Read the model definition and answer for the solid it produces. Units are mm, in the model's axes. Face numbers are marked on the shaded views. Coordinates: 2 decimals unless noted, no trailing zeros. Order: outer loops, then holes, each group sorted by start corner. A loop starts at its lowest first (then second) coordinate and runs counter-clockwise, first axis right, second up.
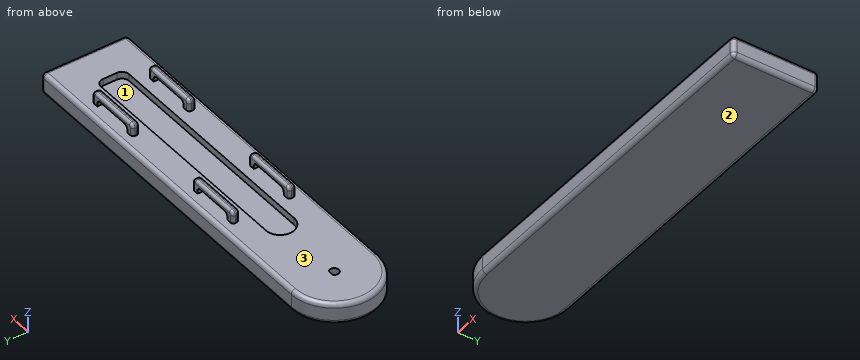
```python
from build123d import *

# Parameters (mm, degrees)
BOSS_EXTRUDE1_DEPTH               = 15
CONG_2_R                          = 3
ENL_V_MAT_EXTRU_3_DEPTH           = 10
BOSS_EXTRU_1_DEPTH                = 5
CONG_3_R                          = 3
CONG_4_R                          = 3
R_P_TITION_LIN_AIRE1_COUNT        = 2
R_P_TITION_LIN_AIRE1_PITCH        = 100
R_P_TITION_LIN_AIRE2_COUNT        = 2
R_P_TITION_LIN_AIRE2_PITCH        = 40
R_P_TITION_LIN_AIRE2_COPY_1_DEPTH = 5
CONG_5_R                          = 3
CONG_6_R                          = 3
CONG_7_R                          = 3
CONG_8_R                          = 2
ENL_V_MAT_EXTRU_5_DEPTH           = 5
CONG_10_R                         = 5


with BuildPart() as part:
    # Sketch1 → Boss-Extrude1 (new body)
    with BuildSketch(Plane.XY):
        with BuildLine():
            Line((0, 30.56), (250, 30.56))
            Line((250, 30.56), (250, -30.56))
            Line((250, -30.56), (0, -30.56))
            ThreePointArc((0, -30.56), (-30.56, 0), (0, 30.56))
        make_face()
    extrude(amount=BOSS_EXTRUDE1_DEPTH)

    # Congé2
    cong_2_edges = [part.edges().sort_by_distance(p)[0] for p in [
        (250, 0, 15),
        (125, 30.56, 15),
        (-30.56, 0, 15),
        (125, 30.56, 0),
        (250, 0, 0),
        (125, -30.56, 0),
        (-30.56, 0, 0),
        (125, -30.56, 15),
        (250, 30.56, 7.5),
        (250, -30.56, 7.5),
    ]]
    fillet(cong_2_edges, radius=CONG_2_R)

    # Esquisse5 → Enlèv. mat.-Extru.3 (cut)
    with BuildSketch(Plane.XY.offset(15)):
        with BuildLine():
            Line((-2.024287639, 2.522286838), (1.975712361, 2.522286838))
            ThreePointArc((1.975712361, 2.522286838), (-0.024287639, -3.175712361), (-2.024287639, 2.522286838))
        make_face()
    extrude(amount=-ENL_V_MAT_EXTRU_3_DEPTH, mode=Mode.SUBTRACT)

    # Esquisse9 → Boss.-Extru.1 (add)
    with BuildSketch(Plane(origin=(0, 22.56, 0), x_dir=(1, 0, 0), z_dir=(0, 1, 0))):
        Polygon((70, -15), (70, -23.5), (110, -23.5), (110, -15), (105, -15), (105, -20), (75, -20), (75, -15), align=None)
    boss_extru_1 = extrude(amount=-BOSS_EXTRU_1_DEPTH)

    # Congé3
    cong_3_edges = [part.edges().sort_by_distance(p)[0] for p in [
        (70, 20.06, 23.5),
    ]]
    fillet(cong_3_edges, radius=CONG_3_R)

    # Congé4
    cong_4_edges = [part.edges().sort_by_distance(p)[0] for p in [
        (75, 20.06, 20),
        (105, 20.06, 20),
        (110, 20.06, 23.5),
    ]]
    fillet(cong_4_edges, radius=CONG_4_R)

    # Répétition linéaire1: Boss.-Extru.1 ×2
    with Locations(*[(i * R_P_TITION_LIN_AIRE1_PITCH, 0, 0) for i in range(1, R_P_TITION_LIN_AIRE1_COUNT)]):
        add(boss_extru_1)

    # Répétition linéaire2: Boss.-Extru.1 ×2
    with Locations(*[(0, -i * R_P_TITION_LIN_AIRE2_PITCH, 0) for i in range(1, R_P_TITION_LIN_AIRE2_COUNT)]):
        add(boss_extru_1)

    # Répétition linéaire2 copy 1 sketch → Répétition linéaire2 copy 1 (add)
    with BuildSketch(Plane(origin=(100, -17.44, 0), x_dir=(1, 0, 0), z_dir=(0, 1, 0))):
        Polygon((70, -15), (70, -23.5), (110, -23.5), (110, -15), (105, -15), (105, -20), (75, -20), (75, -15), align=None)
    extrude(amount=-R_P_TITION_LIN_AIRE2_COPY_1_DEPTH)

    # Congé5
    cong_5_edges = [part.edges().sort_by_distance(p)[0] for p in [
        (75, -19.94, 20),
        (105, -19.94, 20),
        (110, -19.94, 23.5),
        (70, -19.94, 23.5),
    ]]
    fillet(cong_5_edges, radius=CONG_5_R)

    # Congé6
    cong_6_edges = [part.edges().sort_by_distance(p)[0] for p in [
        (175, -19.94, 20),
        (205, -19.94, 20),
        (210, -19.94, 23.5),
        (170, -19.94, 23.5),
    ]]
    fillet(cong_6_edges, radius=CONG_6_R)

    # Congé7
    cong_7_edges = [part.edges().sort_by_distance(p)[0] for p in [
        (175, 20.06, 20),
        (205, 20.06, 20),
        (210, 20.06, 23.5),
        (170, 20.06, 23.5),
    ]]
    fillet(cong_7_edges, radius=CONG_7_R)

    # Congé8
    cong_8_edges = [part.edges().sort_by_distance(p)[0] for p in [
        (170, 17.56, 17.75),
        (170, 22.56, 17.75),
        (70, -22.44, 17.75),
        (70, -17.44, 17.75),
        (170, -22.44, 17.75),
        (170, -17.44, 17.75),
        (90, -17.44, 23.5),
        (110, -17.44, 17.75),
        (109.121320344, -17.44, 22.621320344),
        (70.878679656, -17.44, 22.621320344),
        (90, -22.44, 23.5),
        (110, -22.44, 17.75),
        (109.121320344, -22.44, 22.621320344),
        (70.878679656, -22.44, 22.621320344),
        (190, -17.44, 23.5),
        (190, -22.44, 23.5),
        (210, -17.44, 17.75),
        (170.878679656, -17.44, 22.621320344),
        (209.121320344, -17.44, 22.621320344),
        (210, -22.44, 17.75),
        (170.878679656, -22.44, 22.621320344),
        (209.121320344, -22.44, 22.621320344),
        (190, 22.56, 23.5),
        (210, 22.56, 17.75),
        (209.121320344, 22.56, 22.621320344),
        (170.878679656, 22.56, 22.621320344),
        (190, 17.56, 23.5),
        (210, 17.56, 17.75),
        (209.121320344, 17.56, 22.621320344),
        (170.878679656, 17.56, 22.621320344),
        (70, 17.56, 17.75),
        (70, 22.56, 17.75),
        (90, 22.56, 23.5),
        (70.878679656, 22.56, 22.621320344),
        (90, 17.56, 23.5),
        (70.878679656, 17.56, 22.621320344),
        (110, 22.56, 17.75),
        (109.121320344, 22.56, 22.621320344),
        (110, 17.56, 17.75),
        (109.121320344, 17.56, 22.621320344),
    ]]
    fillet(cong_8_edges, radius=CONG_8_R)

    # Esquisse11 → Enlèv. mat.-Extru.5 (cut)
    with BuildSketch(Plane.XY.offset(15)):
        with BuildLine():
            Line((54, 10.06), (224, 10.06))
            Line((224, 10.06), (224, -9.94))
            Line((224, -9.94), (54, -9.94))
            ThreePointArc((54, -9.94), (44, 0.06), (54, 10.06))
        make_face()
    extrude(amount=-ENL_V_MAT_EXTRU_5_DEPTH, mode=Mode.SUBTRACT)

    # Congé10
    cong_10_edges = [part.edges().sort_by_distance(p)[0] for p in [
        (224, 10.06, 12.5),
        (224, -9.94, 12.5),
    ]]
    fillet(cong_10_edges, radius=CONG_10_R)


solid = part.part
```
1) A cutting plane is placed at B-B, the plane y = 0. Determine the outline of the cut face in (x, z).
A:
outline: (-30.56, 3) arc R3 ccw to (-27.56, 0) - (247, 0) arc R3 ccw to (250, 3) - (250, 12) arc R3 ccw to (247, 15) - (224, 15) - (224, 10) - (44, 10) - (44, 15) - (3.18, 15) - (3.18, 5) - (-3.22, 5) - (-3.22, 15) - (-27.56, 15) arc R3 ccw to (-30.56, 12) - close
2) Flat-ended cylindrical pins translate along their axes: pin 1 Ø1 at (y, z) = (-19.5, 16) entering from +X; pin 2 Ø4 at (x, y) = (115, 4.5) entering from +Z; pin 3 Ø3 at (y, z) = (-6, 17.5) entering from +X; pin 4 Ø1.6 at (y, z) = (-20, 15.5) entering from +X. Find the tip coordinate at first contact, or state that the pin passes through.
A:
pin 1: stops at x = 210
pin 2: stops at z = 10
pin 3: passes through
pin 4: stops at x = 248.31
3) Straight lines are drawn through the part: line 1 (Y direction, x = 173, z = 20); line 2 (Z direction, x = 24, y = 15); line 3 (Y direction, x = 186.5, z = 10.25). For each, find the intervals that lie inside material, in ascending order.
A:
line 1: y = -22.44 to -17.44, 17.56 to 22.56
line 2: z = 0 to 15
line 3: y = -30.56 to -9.94, 10.06 to 30.56
4) Determine the mould class of the marked faces 1, 2 and 3 for opening direction X: pulls with the +X half, pulls with the -X half, needs draft (parallel to the pull), parting line crosses it, or undercut.
A:
face 1: undercut
face 2: needs draft
face 3: undercut
5) A cutting plane is placed at A-A, the plane x = 157. Determine the outline of the cut face in (y, z).
A:
outline: (-30.56, 3) arc R3 ccw to (-27.56, 0) - (27.56, 0) arc R3 ccw to (30.56, 3) - (30.56, 12) arc R3 ccw to (27.56, 15) - (10.06, 15) - (10.06, 10) - (-9.94, 10) - (-9.94, 15) - (-27.56, 15) arc R3 ccw to (-30.56, 12) - close
